from build123d import *

# Parameters (mm, degrees)
BOSS_EXTRUDE1_DEPTH = 1340
CUT_EXTRUDE1_DEPTH  = 1342.082853518


with BuildPart() as part:
    # Sketch1 → Boss-Extrude1 (new body)
    with BuildSketch(Plane.XY):
        with BuildLine():
            Line((2.54, 0), (35.56, 0))
            ThreePointArc((35.56, 0), (37.356051224, -0.743948776), (38.1, -2.54))
            Line((38.1, -2.54), (38.1, -35.56))
            ThreePointArc((38.1, -35.56), (37.356051224, -37.356051224), (35.56, -38.1))
            Line((35.56, -38.1), (2.54, -38.1))
            ThreePointArc((2.54, -38.1), (0.743948776, -37.356051224), (0, -35.56))
            Line((0, -35.56), (0, -2.54))
            ThreePointArc((0, -2.54), (0.743948776, -0.743948776), (2.54, 0))
        make_face()
        with BuildLine():
            Line((5.3086, -2.7686), (32.7914, -2.7686))
            ThreePointArc((32.7914, -2.7686), (34.587451224, -3.512548776), (35.3314, -5.3086))
            Line((35.3314, -5.3086), (35.3314, -32.7914))
            ThreePointArc((35.3314, -32.7914), (34.587451224, -34.587451224), (32.7914, -35.3314))
            Line((32.7914, -35.3314), (5.3086, -35.3314))
            ThreePointArc((5.3086, -35.3314), (3.512548776, -34.587451224), (2.7686, -32.7914))
            Line((2.7686, -32.7914), (2.7686, -5.3086))
            ThreePointArc((2.7686, -5.3086), (3.512548776, -3.512548776), (5.3086, -2.7686))
        make_face(mode=Mode.SUBTRACT)
    extrude(amount=BOSS_EXTRUDE1_DEPTH)

    # Sketch2 → Cut-Extrude1 (cut, through all)
    with BuildSketch(Plane.ZY):
        Polygon((0, -2.54), (5.15810206, -2.54), (5.951656223, 0), (0, 0), align=None)
        Polygon((0, -2.54), (0, -19.05), (5.15810206, -2.54), align=None)
        Polygon((52.845038121, -35.56), (0, -19.05), (0, -35.56), align=None)
        Polygon((60.975043986, -38.1), (52.845038121, -35.56), (0, -35.56), (0, -38.1), align=None)
    extrude(amount=-CUT_EXTRUDE1_DEPTH, mode=Mode.SUBTRACT)


solid = part.part
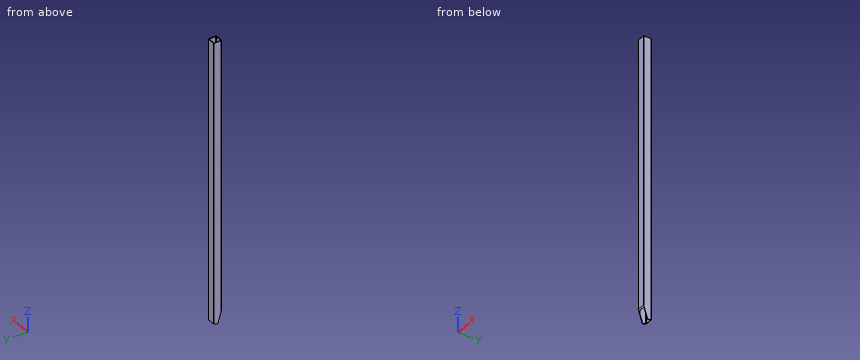
Check sheet for the modelled part. Datum: model origin and axes. Units: mm. Coordinates: 2 decimals unless noted, no trailing zeros. Loops run counter-clockwise (first coordinate to the right, second up) from the corner with the lowest first, then second, coordinate; pieces in that order, holes last. Notation, with made-up numbers: (54, 58) -> (101, 58) arc R21 ccw to (101, 72) -> close; hole circle Ø11 at (60.25, 76). An arc over 180 degrees is marked (long way). Answer in a Markdown table with one row per item.
1. Sectioned sample at B-B, the plane z = 1050.5. Record the boundary of the cut face in (x, y).
Check values:
| item | result |
|---|---|
| outline | (0, -35.56) arc R2.54 ccw to (2.54, -38.1) -> (35.56, -38.1) arc R2.54 ccw to (38.1, -35.56) -> (38.1, -2.54) arc R2.54 ccw to (35.56, 0) -> (2.54, 0) arc R2.54 ccw to (0, -2.54) -> close; hole (2.77, -32.79) arc R2.54 ccw to (5.31, -35.33) -> (32.79, -35.33) arc R2.54 ccw to (35.33, -32.79) -> (35.33, -5.31) arc R2.54 ccw to (32.79, -2.77) -> (5.31, -2.77) arc R2.54 ccw to (2.77, -5.31) -> close |
2. Sectioned sample at A-A, the plane x = 16. Record the boundary of the cut face in (y, z), then the cut area to 3 significant figures.
Check values:
| item | result |
|---|---|
| outline | (-38.1, 60.98) -> (-35.33, 52.11) -> (-35.33, 1340) -> (-38.1, 1340) -> close; (-2.77, 5.09) -> (0, 5.95) -> (0, 1340) -> (-2.77, 1340) -> close |
| area | 7,250 mm2 |
3. Go/stop test with a flat-tipped pin: pin 1 (12 mm diameter, centred on y = -25, z = 427, fed in from -X). Record where the tip stops, or that it passes through.
Check values:
| item | result |
|---|---|
| pin 1 | stops at x = 0 |
4. Material ranges on line 1 along Y through (x, z) = (6, 658.5); line 2 along X through (y, z) = (-28.5, 544); line 3 along Y through (x, z) = (35, 968), recorded low to high. Write a range as [from, to].
Check values:
| item | result |
|---|---|
| line 1 | y = [-38.1, -35.33], [-2.77, 0] |
| line 2 | x = [0, 2.77], [35.33, 38.1] |
| line 3 | y = [-38.1, -34.05], [-4.05, 0] |
